from build123d import *

# Parameters (mm, degrees)
EXTRUDE_1_DEPTH          = 211
SHELL_1_T                = 10
CUT_EXTRUDE_5_REACH      = 317.997
SKETCH_4_R               = 10
CUT_EXTRUDE_6_REACH      = 317.997
SKETCH_5_R               = 10
CUT_EXTRUDE_9_DEPTH      = 316.997319763
CUT_EXTRUDE_9_DEPTH_BACK = 316.997319763


with BuildPart() as part:
    # 草图1 → 凸台-拉伸1 (new body)
    with BuildSketch(Plane.XY):
        Polygon((122, 0), (-122, 0), (-179.100687039, 98.901291098), (-86.265, 152.5), (86.265, 152.5), (179.100687039, 98.901291098), align=None)
    extrude(amount=EXTRUDE_1_DEPTH)

    # 抽壳1 (no face opened: a closed hollow body)
    add(offset(amount=-SHELL_1_T, mode=Mode.PRIVATE), mode=Mode.SUBTRACT)

    # 草图4 → 切除-拉伸5 (cut, up to next)
    with BuildSketch(Plane(origin=(0, 0, 0), x_dir=(-1, 0, 0), z_dir=(0, 0, -1)), mode=Mode.PRIVATE) as cut_extrude_5_sk1:
        with Locations((-54.9, 36.6)):
            Circle(SKETCH_4_R)
    cut_extrude_5_tool1 = extrude(cut_extrude_5_sk1.sketch, amount=-CUT_EXTRUDE_5_REACH, mode=Mode.PRIVATE) & part.part
    # 草图4 → 切除-拉伸5 (cut, up to next)
    with BuildSketch(Plane(origin=(0, 0, 0), x_dir=(-1, 0, 0), z_dir=(0, 0, -1)), mode=Mode.PRIVATE) as cut_extrude_5_sk2:
        with Locations((54.9, 36.6)):
            Circle(SKETCH_4_R)
    cut_extrude_5_tool2 = extrude(cut_extrude_5_sk2.sketch, amount=-CUT_EXTRUDE_5_REACH, mode=Mode.PRIVATE) & part.part
    add(cut_extrude_5_tool1.solids().sort_by_distance((54.9, 36.6, 0))[0], mode=Mode.SUBTRACT)
    add(cut_extrude_5_tool2.solids().sort_by_distance((-54.9, 36.6, 0))[0], mode=Mode.SUBTRACT)

    # 草图5 → 切除-拉伸6 (cut, up to next)
    with BuildSketch(Plane.XY.offset(211), mode=Mode.PRIVATE) as cut_extrude_6_sk1:
        with Locations((-72.089123196, 122)):
            Circle(SKETCH_5_R)
    cut_extrude_6_tool1 = extrude(cut_extrude_6_sk1.sketch, amount=-CUT_EXTRUDE_6_REACH, mode=Mode.PRIVATE) & part.part
    # 草图5 → 切除-拉伸6 (cut, up to next)
    with BuildSketch(Plane.XY.offset(211), mode=Mode.PRIVATE) as cut_extrude_6_sk2:
        with Locations((74.310876804, 120.659584251)):
            Circle(SKETCH_5_R)
    cut_extrude_6_tool2 = extrude(cut_extrude_6_sk2.sketch, amount=-CUT_EXTRUDE_6_REACH, mode=Mode.PRIVATE) & part.part
    add(cut_extrude_6_tool1.solids().sort_by_distance((-72.089123, 122, 211))[0], mode=Mode.SUBTRACT)
    add(cut_extrude_6_tool2.solids().sort_by_distance((74.310877, 120.659584, 211))[0], mode=Mode.SUBTRACT)

    # 草图7 → 切除-拉伸9 (cut, two sides: drawn at the far end of the back side and taken through both)
    with BuildSketch(Plane(origin=(0, 0, 0), x_dir=(0, 0, -1), z_dir=(1, 0, 0)).offset(-CUT_EXTRUDE_9_DEPTH_BACK)):
        Polygon((0, 73.2), (-201, 95.24103706), (-201, 152.5), (0, 152.5), align=None)
    extrude(amount=CUT_EXTRUDE_9_DEPTH + CUT_EXTRUDE_9_DEPTH_BACK, mode=Mode.SUBTRACT)


solid = part.part
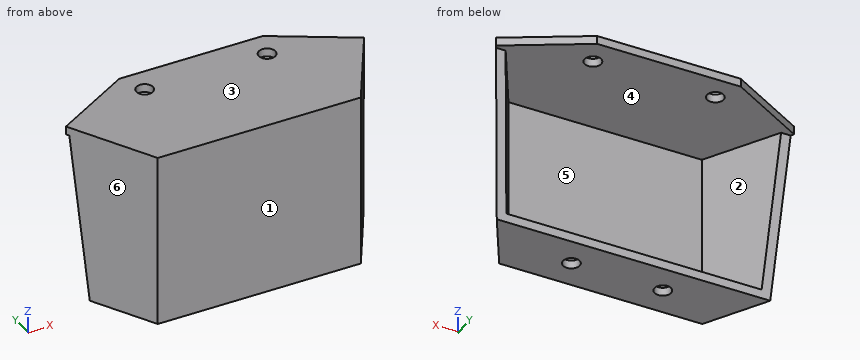
Can you work these out from the model? Positions are in its coordinate system, mm. Face numbers are marked on the shaded views. A direction names the side the tool comes from. Coordinates: 2 decimals unless noted, no trailing zeros. Write each loop counter-clockwise with the first axis right and the second up, starting at its lowest first coordinate (ties: lowest second). Pieces come first, ordered by that corner, then holes.
Q1. For P1, Ø10, axis at x = -140, y = 75, coming from the -Z side; P2, Ø10, axis at y = 38, z = 126, coming from the +X side; P3, Ø1.5, axis at x = 140, z = 138, coming from the -Y side; P4, Ø4, axis at x = 115.5, z = 83.5, coming from the +Y side, each with a flat end and sliding along its axis, tell me the tip position at first contact or that it passes through.
Results found:
P1: stops at z = 0
P2: stops at x = 146.83
P3: stops at y = 29.88
P4: stops at y = 12.21
Q2. Imagine slicing it at A-A, the plane x = 54.9. List the corners of the cut face in (y, z) for me.
Results found:
outline: (0, 0) - (26.6, 0) - (26.6, 10) - (10, 10) - (10, 201) - (152.5, 201) - (152.5, 211) - (0, 211) - close; (46.6, 0) - (73.2, 0) - (74.3, 10) - (46.6, 10) - close
Q3. Imagine slicing it at D-D, the plane y = 36.6. List the corners of the cut face in (x, z) for me, plus the area to 3 significant figures.
Results found:
outline: (-143.13, 0) - (-64.9, 0) - (-64.9, 10) - (-131.58, 10) - (-131.58, 201) - (131.58, 201) - (131.58, 10) - (64.9, 10) - (64.9, 0) - (143.13, 0) - (143.13, 211) - (-143.13, 211) - close; (-44.9, 0) - (44.9, 0) - (44.9, 10) - (-44.9, 10) - close
area: 9,740 mm2
Q4. Imagine slicing it at B-B, the plane x = -24. List the corners of the cut face in (y, z) for me.
Results found:
outline: (0, 0) - (73.2, 0) - (74.3, 10) - (10, 10) - (10, 201) - (152.5, 201) - (152.5, 211) - (0, 211) - close
Q5. Please list where these lines run through material, in increasing order: L1, parallel to Z at x = -34.5, y = 20.5; L2, parallel to X at y = 36, z = 7; L3, parallel to Y at x = 41.5, z = 84.5.
Results found:
L1: z = 0 to 10, 201 to 211
L2: x = -142.78 to -64.88, -44.92 to 44.92, 64.88 to 142.78
L3: y = 0 to 10
Q6. Imagine slicing it at C-C, the plane z = 153. List the corners of the cut face in (x, y) for me.
Results found:
outline: (-173.95, 89.98) - (-122, 0) - (122, 0) - (173.95, 89.98) - (162.4, 89.98) - (116.23, 10) - (-116.23, 10) - (-162.4, 89.98) - close
Q7. If we mould it in two halves opening along Z, with no side actions, what happens to the marked faces 1, 2, 3 and 4? For each: +Z half, -Z half, draft (parallel to the pull), parting line (faces both ways), or undercut.
Results found:
face 1: draft
face 2: undercut
face 3: +Z half
face 4: undercut
Q8. Which directions (+Z, -Z, +X, -X, +Y, -Y) give clear straight access to the entire face, cutting with the end or side of a thin tool? Please do the marked faces 5 and 6.
Results found:
face 5: +Y
face 6: +Z, -Z, -X, -Y
